Read the model definition and answer for the solid it produces. Units are mm, in the model's axes. Face numbers are marked on the shaded views. A direction names the side the tool comes from. Round coordinates to 2 decimals unless told otherwise and drop trailing zeros. Order: outer loops, then holes, each group sorted by start corner. A loop starts at its lowest first (then second) coordinate and runs counter-clockwise, first axis right, second up. Notation, with made-up numbers: (56, 64) - (72, 64) arc R16 ccw to (72, 82) - close; hole circle Ø10 at (58.25, -6). An arc over 180 degrees is marked (long way). Answer as a JSON object with one key per item and string values. Group by question number.
Q1. The mould has two halves that part along X. Classify the marked faces 3, 4 and 5: pulls with the +X half, pulls with the -X half, needs draft (parallel to the pull), parting line crosses it, or undercut.
Q2. A cutting plane is placed at A-A on y = 0. Determine the outline of the cut face in (x, z), and give its area (3 significant figures).
Q3. Given pin 1 Ø4 at (x, y) = (57.5, -42.5) entering from -Z; pin 2 Ø1 at (y, z) = (-24.5, -16.5) entering from -X; pin 3 Ø2 at (y, z) = (-10.5, -21.5) entering from -X, each flat-ended and moving along its own axis, determine where each tip first touches the part or whether it passes through.
Q4. A tool of negligible diameter and unlimited length cuts with its end or side. For the marked faces 1 and 2, from which of +Z, -Z, +X, -X, +Y, -Y can it reach the whole face along a straight path? Write none if from no direction.
Q5. A cutting plane is placed at B-B on z = -22. Determine the outline of the cut face in (x, y), and give its area (3 significant figures).
Q6. Consider line 1 (Y direction, x = 57.5, z = 1.25); line 2 (Y direction, x = -42.5, z = 2.35); line 3 (Y direction, x = 36, z = 2.3). Determine where each line is inside the solid, lowest interval first.
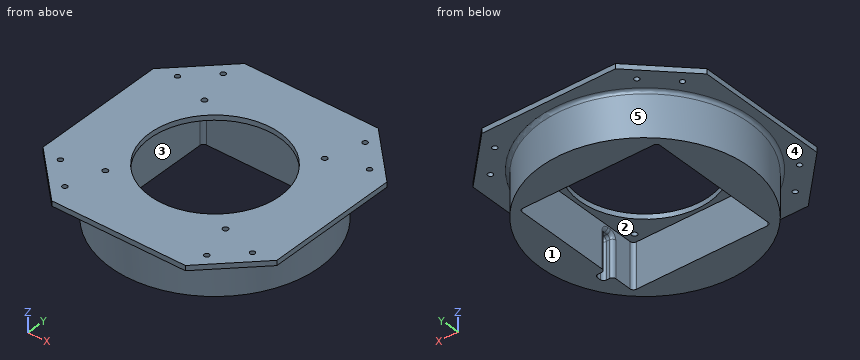
```python
from build123d import *

# Parameters (mm, degrees)
SKETCH_W        = 140
SKETCH_H        = 140
PAD_DEPTH       = 3
SKETCH001_R     = 62.5
PAD001_DEPTH    = 27
SKETCH002_W     = 82.5
SKETCH002_H     = 82.5
POCKET_DEPTH    = 27
SKETCH003_R     = 1.6
SKETCH003_R_2   = 39
POCKET001_DEPTH = 5
FILLET_R        = 2
CHAMFER_SIZE    = 30
SKETCH004_R     = 1.5
HOLE_DEPTH      = 25
SKETCH005_W     = 6
SKETCH005_H     = 6
POCKET002_DEPTH = 24
FILLET001_R     = 2
FILLET002_R     = 2


with BuildPart() as part:
    # Sketch → Pad (new body)
    with BuildSketch(Plane.XY):
        Rectangle(SKETCH_W, SKETCH_H)
    extrude(amount=PAD_DEPTH)

    # Sketch001 (on Face5 of Pad) → Pad001 (join)
    with BuildSketch(Plane(origin=(0, 0, 0), x_dir=(1, 0, 0), z_dir=(0, 0, -1))):
        Circle(SKETCH001_R)
    extrude(amount=PAD001_DEPTH)

    # Sketch002 (on Face8 of Pad001) → Pocket (cut)
    with BuildSketch(Plane(origin=(0, 0, -27), x_dir=(1, 0, 0), z_dir=(0, 0, -1))):
        Rectangle(SKETCH002_W, SKETCH002_H)
    extrude(amount=-POCKET_DEPTH, mode=Mode.SUBTRACT)

    # Sketch003 (on Face13 of Pocket) → Pocket001 (cut)
    with BuildSketch(Plane(origin=(0, 0, 0), x_dir=(1, 0, 0), z_dir=(0, 0, -1))):
        with Locations((-36, 36)):
            Circle(SKETCH003_R)
        with Locations((36, 36)):
            Circle(SKETCH003_R)
        with Locations((-36, -36)):
            Circle(SKETCH003_R)
        with Locations((36, -36)):
            Circle(SKETCH003_R)
        Circle(SKETCH003_R_2)
    extrude(amount=-POCKET001_DEPTH, mode=Mode.SUBTRACT)

    # Fillet
    fillet_edges = [part.edges().sort_by_distance(p)[0] for p in [
        (41.25, 41.25, -13.5),
        (-41.25, 41.25, -13.5),
        (-41.25, -41.25, -13.5),
        (41.25, -41.25, -13.5),
    ]]
    fillet(fillet_edges, radius=FILLET_R)

    # Chamfer
    chamfer_edges = [part.edges().sort_by_distance(p)[0] for p in [
        (70, 70, 1.5),
        (-70, 70, 1.5),
        (70, -70, 1.5),
        (-70, -70, 1.5),
    ]]
    chamfer(chamfer_edges, length=CHAMFER_SIZE)

    # Sketch004 (on Face1 of Chamfer) → Hole (cut)
    with BuildSketch(Plane(origin=(0, 0, 0), x_dir=(1, 0, 0), z_dir=(0, 0, -1))):
        with Locations((-42.5, 57.5)):
            Circle(SKETCH004_R)
        with Locations((-57.5, 42.5)):
            Circle(SKETCH004_R)
        with Locations((42.5, 57.5)):
            Circle(SKETCH004_R)
        with Locations((57.5, 42.5)):
            Circle(SKETCH004_R)
        with Locations((57.5, -42.5)):
            Circle(SKETCH004_R)
        with Locations((42.5, -57.5)):
            Circle(SKETCH004_R)
        with Locations((-42.5, -57.5)):
            Circle(SKETCH004_R)
        with Locations((-57.5, -42.5)):
            Circle(SKETCH004_R)
    extrude(amount=-HOLE_DEPTH, mode=Mode.SUBTRACT)

    # Sketch005 (on Face20 of Hole) → Pocket002 (cut)
    with BuildSketch(Plane(origin=(0, 0, -27), x_dir=(1, 0, 0), z_dir=(0, 0, -1))):
        with Locations((44.25, 23.811943)):
            Rectangle(SKETCH005_W, SKETCH005_H)
    extrude(amount=-POCKET002_DEPTH, mode=Mode.SUBTRACT)

    # Fillet001
    fillet001_edges = [part.edges().sort_by_distance(p)[0] for p in [
        (41.25, -26.811943, -15),
        (47.25, -26.811943, -15),
        (47.25, -20.811943, -15),
        (41.25, -20.811943, -15),
        (44.25, -26.811943, -3),
        (47.25, -23.811943, -3),
        (44.25, -20.811943, -3),
        (41.25, -23.811943, -3),
    ]]
    fillet(fillet001_edges, radius=FILLET001_R)

    # Fillet002
    fillet002_edges = [part.edges().sort_by_distance(p)[0] for p in [
        (-62.5, 0, 0),
    ]]
    fillet(fillet002_edges, radius=FILLET002_R)


solid = part.part
```
Result set:
{
 "1": {"face 3": "undercut", "face 4": "needs draft", "face 5": "parting line crosses it"},
 "2": {"outline": "(-70, 0) - (-64.5, 0) arc R2 cw to (-62.5, -2) - (-62.5, -27) - (-41.25, -27) - (-41.25, 0) - (-39, 0) - (-39, 3) - (-70, 3) - close; (39, 0) - (41.25, 0) - (41.25, -27) - (62.5, -27) - (62.5, -2) arc R2 cw to (64.5, 0) - (70, 0) - (70, 3) - (39, 3) - close", "area": "1,340 mm²"},
 "3": {"pin 1": "stops at z = 0", "pin 2": "stops at x = -57.71", "pin 3": "stops at x = -61.77"},
 "4": {"face 1": "-Z, +X, -X, +Y, -Y", "face 2": "-Z"},
 "5": {"outline": "circle Ø125 at (0, 0); hole (-41.25, -39.25) arc R2 ccw to (-39.25, -41.25) - (39.25, -41.25) arc R2 ccw to (41.25, -39.25) - (41.25, -28.81) arc R2 cw to (43.25, -26.81) - (45.25, -26.81) arc R2 ccw to (47.25, -24.81) - (47.25, -22.81) arc R2 ccw to (45.25, -20.81) - (43.25, -20.81) arc R2 cw to (41.25, -18.81) - (41.25, 39.25) arc R2 ccw to (39.25, 41.25) - (-39.25, 41.25) arc R2 ccw to (-41.25, 39.25) - close", "area": "5,430 mm²"},
 "6": {"line 1": "y = -52.5 to -44, -41 to 41, 44 to 52.5", "line 2": "y = -67.5 to -59, -56 to 56, 59 to 67.5", "line 3": "y = -70 to -37.6, -34.4 to -15, 15 to 34.4, 37.6 to 70"}
}
